For this review, take the finished solid that the model builds, in its own axes (mm). Round coordinates to 2 decimals unless told otherwise and drop trailing zeros. Order: outer loops, then holes, each group sorted by start corner. A loop starts at its lowest first (then second) coordinate and runs counter-clockwise, first axis right, second up. Notation, with made-up numbers: (-37, 9) -> (7, 9) arc R31 ccw to (7, 42) -> close; hole circle Ø4 at (44, 71.25). An arc over 180 degrees is marked (long way). Use a Markdown table: item, result. Add a question column.
1) Draft analysis for pull direction Y (two halves, no side actions). For faces 1 (the face through (-10, 0, 1)), 2 (the face through (0, 25, 1)), 3 (the face through (-0.56, -10.46, 0.99)), state which applies: pulls with the +Y half, pulls with the -Y half, needs draft (parallel to the pull), parting line crosses it, or undercut.
2) Wall thickness on line 1 along Y through (x, z) = (0, 1.55); line 2 along Y through (x, z) = (2, 0.45); line 3 along X through (y, z) = (16.5, 0.5): over which ranges is each line inside the solid? List them lowest first. Write a range as [from, to].
3) Consider section D-D (x = 2). State the section outline as (y, z) points, plus the area to 3 significant figures.
4) Clearance check with a flat-ended pin moving along its axis: P1, Ø6, axis at x = 0, y = -13, coming from the +Z side. State where the tip first meets the part, or that it passes through.
5) Consider section A-A (y = -13). State the section outline as (x, z) points, plus the area to 3 significant figures.
6) Consider section B-B (x = 0). State the section outline as (y, z) points, plus the area to 3 significant figures.
7) Consider section C-C (z = 0.6). State the section outline as (x, y) points, plus the area to 3 significant figures.
Autodesk Inventor part; units mm, degrees
ref_plane "YZ Plane" through (0, 0, 0) normal (1, 0, 0) x (0, 1, 0)
ref_plane "XZ Plane" through (0, 0, 0) normal (0, 1, 0) x (-1, 0, 0)
ref_plane "XY Plane" through (0, 0, 0) normal (0, 0, 1) x (1, 0, 0)
sketch "Sketch1" plane through (0, 0, 0) normal (0, 0, 1) x (1, 0, 0)
  line L0 (-10, 25) -> (10, 25)
  line L1 (10, 25) -> (10, -25)
  line L2 (10, -25) -> (-10, -25)
  line L3 (-10, -25) -> (-10, 25)
  circle A0 centre (0, -13) radius 2.6
  circle A1 centre (0, 18) radius 3.1
  point P0 (0, 0)
  dimension "d0" = 20
  dimension "d1" = 50
  dimension "d2" = 5.2
  dimension "d3" = 6.2
extrude "Extrusion1" add sketch "Sketch1" along normal blind 2
properties part number "Bed Plate Hang"
Results list:
| question | item | result |
|---|---|---|
| 1 | face 1 | needs draft |
| 1 | face 2 | pulls with the +Y half |
| 1 | face 3 | undercut |
| 2 | line 1 | [-25, -15.6], [-10.4, 14.9], [21.1, 25] |
| 2 | line 2 | [-25, -14.66], [-11.34, 15.63], [20.37, 25] |
| 2 | line 3 | [-10, -2.71], [2.71, 10] |
| 3 | outline | (-25, 0) -> (-14.66, 0) -> (-14.66, 2) -> (-25, 2) -> close; (-11.34, 0) -> (15.63, 0) -> (15.63, 2) -> (-11.34, 2) -> close; (20.37, 0) -> (25, 0) -> (25, 2) -> (20.37, 2) -> close |
| 3 | area | 83.9 mm2 |
| 4 | P1 | z = 2 |
| 5 | outline | (-10, 0) -> (-2.6, 0) -> (-2.6, 2) -> (-10, 2) -> close; (2.6, 0) -> (10, 0) -> (10, 2) -> (2.6, 2) -> close |
| 5 | area | 29.6 mm2 |
| 6 | outline | (-25, 0) -> (-15.6, 0) -> (-15.6, 2) -> (-25, 2) -> close; (-10.4, 0) -> (14.9, 0) -> (14.9, 2) -> (-10.4, 2) -> close; (21.1, 0) -> (25, 0) -> (25, 2) -> (21.1, 2) -> close |
| 6 | area | 77.2 mm2 |
| 7 | outline | (-10, -25) -> (10, -25) -> (10, 25) -> (-10, 25) -> close; hole circle Ø6.2 at (0, 18); hole circle Ø5.2 at (0, -13) |
| 7 | area | 949 mm2 |
